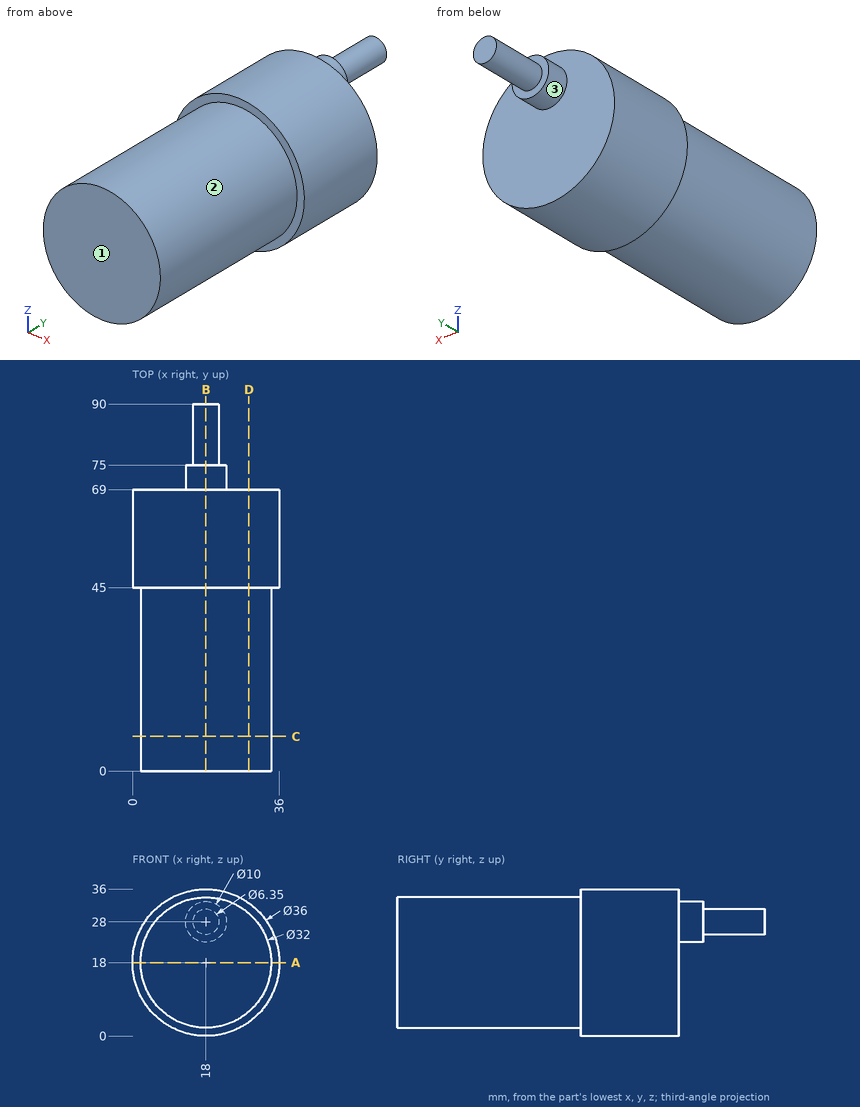
Design review of the part shown in the three views and the two pictorial views. Dimensions are in mm from the part's minimum x, y and z. A direction names the side the tool comes from. Coordinates: 2 decimals unless noted, no trailing zeros. Write each loop counter-clockwise with the first axis right and the second up, starting at its lowest first coordinate (ties: lowest second). Pieces come first, ordered by that corner, then holes.
(1) Wall thickness on probe 1 along Y at (x, z) = (8, 12.5); probe 2 along Z at (x, y) = (17.5, 48); probe 3 along Z at (x, y) = (10.5, 31): over which ranges is each line inside the solid? List them lowest first.
(2) For pin 1 Ø1.5 at (x, y) = (22, 64.5) entering from -Z; pin 2 Ø10 at (x, y) = (31.5, 71) entering from +Z; pin 3 Ø5 at (y, z) = (13, 14) entering from +X, all flat-tipped, find the tip position at first contact; note any pin that passes through.
(3) Tool access review of the marked faces 1, 2 and 3: name each direction out of +Z, -Z, +X, -X, +Y, -Y from which nothing blocks a thin tool from reaching the whole face with its end or side.
(4) Add section C-C on y = 8.5. Give the boundary of the cut face in (x, z).
(5) Add section A-A on z = 18. Give the boundary of the cut face in (x, y).
(6) Add section D-D on x = 28.5. Give the boundary of the cut face in (y, z), then the cut area to 3 significant figures.
(7) Add section B-B on x = 18. Give the boundary of the cut face in (y, z) (3 decimals), then the cut area to 3 significant figures.
Answer sheet:
1. probe 1: y = 0 to 69
1. probe 2: z = 0.01 to 35.99
1. probe 3: z = 3.87 to 32.13
2. pin 1: stops at z = 0.3
2. pin 2: stops at z = 33.64
2. pin 3: stops at x = 33.93
3. face 1: +Z, -Z, +X, -X, -Y
3. face 2: -Y
3. face 3: +Y
4. outline: circle Ø32 at (18, 18)
5. outline: (0, 45) - (2, 45) - (2, 0) - (34, 0) - (34, 45) - (36, 45) - (36, 69) - (0, 69) - close
6. outline: (0, 5.93) - (45, 5.93) - (45, 3.38) - (69, 3.38) - (69, 32.62) - (45, 32.62) - (45, 30.07) - (0, 30.07) - close
6. area: 1,790 mm2
7. outline: (0, 2) - (45, 2) - (45, 0) - (69, 0) - (69, 23) - (75, 23) - (75, 24.825) - (90, 24.825) - (90, 31.175) - (75, 31.175) - (75, 33) - (69, 33) - (69, 36) - (45, 36) - (45, 34) - (0, 34) - close
7. area: 2,460 mm2
